Geometry check sheet. Reference: the model listing, model coordinates, mm. A direction names the side the tool comes from. Coordinates: 2 decimals unless noted, no trailing zeros. Loops run counter-clockwise (first coordinate to the right, second up) from the corner with the lowest first, then second, coordinate; pieces in that order, holes last. Notation, with made-up numbers: (58, 25) -> (67, 25) arc R18 cw to (67, 39) -> close; hole circle Ø4 at (84, 15). An arc over 180 degrees is marked (long way). Answer as a JSON object with one key per item and string values.
from build123d import *

# Parameters (mm, degrees)
CYLINDER2005_R               = 1.5
CYLINDER2005_DEPTH           = 60
CYLINDER2002_R               = 1.5
CYLINDER2002_DEPTH           = 60
CYLINDER2003_R               = 1.5
CYLINDER2003_DEPTH           = 60
CYLINDER2004_R               = 1.5
CYLINDER2004_DEPTH           = 60
COMPOUND1081_PLACEMENT_ANGLE = 225
CYLINDER1969_R               = 74
CYLINDER1969_DEPTH           = 40
BOX980_W                     = 42
BOX980_H                     = 72
BOX980_DEPTH                 = 50
COMPOUND1061_PLACEMENT_ANGLE = 225
BOX981_W                     = 54
BOX981_H                     = 78
BOX981_DEPTH                 = 9
COMPOUND1062_PLACEMENT_ANGLE = 225
CHAMFER072_SIZE              = 3


with BuildPart() as obj1:
    # Cylinder2005 → Cylinder2005 (new body)
    with BuildSketch(Plane(origin=(-24, 74, -80), x_dir=(1, 0, 0), z_dir=(0, 0, 1))):
        Circle(CYLINDER2005_R)
    extrude(amount=CYLINDER2005_DEPTH)


with BuildPart() as obj2:
    # Cylinder2002 → Cylinder2002 (new body)
    with BuildSketch(Plane(origin=(-15, 135, -80), x_dir=(1, 0, 0), z_dir=(0, 0, 1))):
        Circle(CYLINDER2002_R)
    extrude(amount=CYLINDER2002_DEPTH)


with BuildPart() as obj3:
    # Cylinder2003 → Cylinder2003 (new body)
    with BuildSketch(Plane(origin=(15, 135, -80), x_dir=(1, 0, 0), z_dir=(0, 0, 1))):
        Circle(CYLINDER2003_R)
    extrude(amount=CYLINDER2003_DEPTH)


with BuildPart() as compound1081:
    # Cylinder2004 → Cylinder2004 (new body)
    with BuildSketch(Plane(origin=(24, 74, -80), x_dir=(1, 0, 0), z_dir=(0, 0, 1))):
        Circle(CYLINDER2004_R)
    extrude(amount=CYLINDER2004_DEPTH)

    # Compound1081: union obj1, obj2, obj3
    add(obj1.part)
    add(obj2.part)
    add(obj3.part)


with BuildPart() as compound1081_1:
    # Compound1081 placement: moved
    add(compound1081.part.moved(Location((0, 0, 109))).rotate(Axis((0, 0, 109), (0, 0, 1)), COMPOUND1081_PLACEMENT_ANGLE))


with BuildPart() as obj4:
    # Cylinder1969 → Cylinder1969 (new body)
    with BuildSketch(Plane.XY.offset(44)):
        Circle(CYLINDER1969_R)
    extrude(amount=CYLINDER1969_DEPTH)


with BuildPart() as compound1061:
    # Box980 → Box980 (new body)
    with BuildSketch(Plane(origin=(-21.001071, 60.005081, 31), x_dir=(1, 0, 0), z_dir=(0, 0, 1))):
        with Locations((21, 36)):
            Rectangle(BOX980_W, BOX980_H)
    extrude(amount=BOX980_DEPTH)


with BuildPart() as compound1061_1:
    # Compound1061 placement: moved
    add(compound1061.part.moved(Location((0, 0, 1))).rotate(Axis((0, 0, 1), (0, 0, 1)), COMPOUND1061_PLACEMENT_ANGLE))


with BuildPart() as cut677:
    # Box981 → Box981 (new body)
    with BuildSketch(Plane(origin=(-27.004408, 59.99801, 75), x_dir=(1, 0, 0), z_dir=(0, 0, 1))):
        with Locations((27, 39)):
            Rectangle(BOX981_W, BOX981_H)
    extrude(amount=BOX981_DEPTH)


with BuildPart() as cut677_1:
    # Compound1062 placement: moved
    add(cut677.part.rotate(Axis((0, 0, 0), (0, 0, 1)), COMPOUND1062_PLACEMENT_ANGLE))

    # Cut662: cut Compound1061
    add(compound1061_1.part, mode=Mode.SUBTRACT)

    # Cut663: cut obj4
    add(obj4.part, mode=Mode.SUBTRACT)

    # Chamfer072
    chamfer072_edges = [cut677_1.edges().sort_by_distance(p)[0] for p in [
        (116.674329, -78.484329, 79.5),
        (78.490563, -116.668095, 79.5),
    ]]
    chamfer(chamfer072_edges, length=CHAMFER072_SIZE)

    # Cut677: cut Compound1081
    add(compound1081_1.part, mode=Mode.SUBTRACT)


solid = cut677_1.part
1. Section check B-B, the plane x = 74. Record the boundary of the cut face in (y, z).
Evaluation:
{"outline": "(-112.18, 75) -> (-103.7, 75) -> (-103.7, 82) -> (-44.3, 82) -> (-44.3, 75) -> (-35.81, 75) -> (-35.81, 84) -> (-112.18, 84) -> close"}
2. Section check A-A, the plane y = -88. Record the boundary of the cut face in (x, z).
Evaluation:
{"outline": "(49.82, 75) -> (58.3, 75) -> (58.3, 82) -> (98.68, 82) -> (98.68, 75) -> (107.16, 75) -> (107.16, 84) -> (49.82, 84) -> close"}
3. Thickness scan on probe 1 along X at (y, z) = (-68, 77); probe 2 along Z at (x, y) = (74, -80); probe 3 along Y at (x, z) = (69, 78.5). Record the ranges inside material, lowest first. Write a range as from..to.
Evaluation:
{"probe 1": "x = 29.82..34.6, 36.11..38.3, 97.7..106.19", "probe 2": "z = 82..84", "probe 3": "y = -107.18..-98.7, -39.3..-36.83, -33.88..-30.81"}
4. Section check C-C, the plane z = 79.5. Record the boundary of the cut face in (x, y).
Evaluation:
{"outline": "(29.63, -67.81) -> (76.37, -114.55) -> (80.61, -114.55) -> (114.55, -80.61) -> (114.55, -76.36) -> (67.81, -29.62) arc R74 cw to (65.02, -35.32) -> (108.19, -78.49) -> (78.49, -108.19) -> (35.33, -65.02) arc R74 cw to start; hole circle Ø3 at (35.36, -69.3); hole circle Ø3 at (69.3, -35.36); hole circle Ø3 at (84.85, -106.07); hole circle Ø3 at (106.07, -84.85)"}
5. Tool access check on faces 5 (the face through (93.55, -93.133, 78.451)), 6 (the face through (90.86, -52.67, 79.44)). Record the directions out of +Z, -Z, +X, -X, +Y, -Y that give a thin tool (end or side, any length) a straight path to the whole face; none if there is none.
Evaluation:
{"face 5": "-Z", "face 6": "+Z, -Z, +X, +Y"}
6. Mould release check, pull along Y, two halves, no side actions. Record for faces 1 (the face through (52.67, -90.85, 79.44)), 2 (the face through (36.46, -68.28, 79.44)), 3 (the face through (52.05, -52.6, 82.44)), 4 (the face through (56.608, -86.305, 78.451)): released by +Y, released by -Y, zero draft, split by the parting line, or undercut.
Evaluation:
{"face 1": "released by -Y", "face 2": "undercut", "face 3": "released by +Y", "face 4": "undercut"}
7. Depth check by flat-ended pin: P1, Ø3, axis at x = 88.5, z = 83, coming from the +Y side; P2, Ø3, axis at y = -73, z = 77.5, coming from the -X side; P3, Ø2, axis at x = 55.5, z = 80, coming from the +Y side. Enter the tip coordinate at first touch or a pass-through.
Evaluation:
{"P1": "stops at y = -48.81", "P2": "stops at x = 33.32", "P3": "stops at y = -84.2"}
8. Section check D-D, the plane y = -54. Record the boundary of the cut face in (x, z), then the cut area to 3 significant figures.
Evaluation:
{"outline": "(50.6, 82) -> (83.7, 82) -> (83.7, 75) -> (92.19, 75) -> (92.19, 84) -> (50.6, 84) -> close", "area": "143 mm^2"}
